```python
from build123d import *

# Parameters (mm, degrees)
F1_DEPTH = 25.4


with BuildPart() as f1:
    # F0 (on Front) → F1 (new body)
    with BuildSketch(Plane.XZ):
        with BuildLine():
            Line((0, 26.083848), (0, 0))
            Line((0, 0), (57.15, 0))
            Line((57.15, 0), (57.15, 19.05))
            ThreePointArc((57.15, 19.05), (43.643284, 24.593284), (38.1, 38.1))
            Line((38.1, 38.1), (10.160001, 38.1))
            Line((10.160001, 38.1), (9.190616, 38.1))
            ThreePointArc((9.190616, 38.1), (3.279744, 35.770442), (0, 30.329071))
            Line((0, 30.329071), (0, 26.083848))
        make_face()
    extrude(amount=F1_DEPTH)


solid = f1.part
```
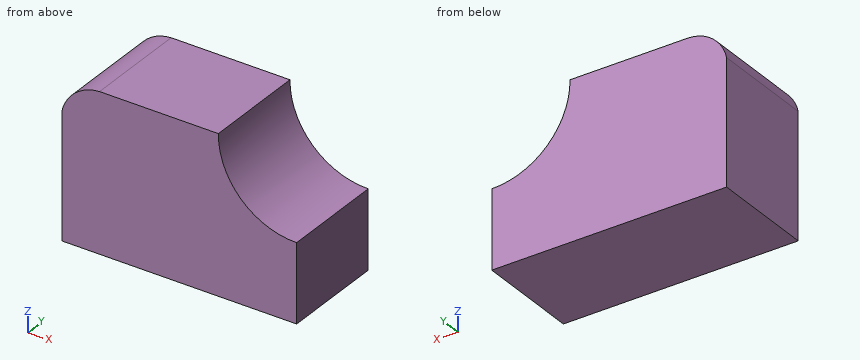
Build history of the part. All positions in model axes, mm. Coordinates: 2 decimals unless noted, no trailing zeros. Write each loop counter-clockwise with the first axis right and the second up, starting at its lowest first coordinate (ties: lowest second). Pieces come first, ordered by that corner, then holes.
1. Drill centre lines: probe 1 along Z at (x, y) = (44, -11.5); probe 2 along X at (y, z) = (-9.75, 24); probe 3 along Z at (x, y) = (8, -17.75). Where is each one in solid material? Low to high.
Answer block:
probe 1: z = 0 to 24.25
probe 2: x = 0 to 44.26
probe 3: z = 0 to 37.97
2. Band-saw the part on B-B, the plane x = 50.5. Give the cut face in (y, z).
Answer block:
outline: (-25.4, 0) - (0, 0) - (0, 20.21) - (-25.4, 20.21) - close
3. Drop flat-ended pins along their axis: pin 1 (3 mm diameter, centred on x = 50.5, y = -6, fed in from +Z); pin 2 (3 mm diameter, centred on y = -15.5, z = 33.5, fed in from -X). Give the stop position or say it passes through.
Answer block:
pin 1: stops at z = 20.84
pin 2: stops at x = 0.53
4. Band-saw the part on C-C, the plane z = 23. Give the cut face in (x, y).
Answer block:
outline: (0, -25.4) - (45.45, -25.4) - (45.45, 0) - (0, 0) - close
5. Band-saw the part on A-A, the plane y = -21. Give the cut face in (x, z), and give its area (3 significant figures).
Answer block:
outline: (0, 0) - (57.15, 0) - (57.15, 19.05) arc R18.93 cw to (38.1, 38.1) - (9.19, 38.1) arc R9.91 ccw to (0, 30.33) - close
area: 1,870 mm2
